```python
from build123d import *

# Parameters (mm, degrees)
EXTRUDE_1_DEPTH     = 10
EXTRUDE_2_DEPTH     = 120
CUT_EXTRUDE_1_DEPTH = 10
EXTRUDE_3_DEPTH     = 10
SKETCH_8_W          = 35
SKETCH_8_H          = 50
EXTRUDE_4_DEPTH     = 50


with BuildPart() as part:
    # 草图1 → 凸台-拉伸1 (new body)
    with BuildSketch(Plane.XY):
        with BuildLine():
            Line((30, 0), (120, 0))
            ThreePointArc((120, 0), (141.213203436, 8.786796564), (150, 30))
            Line((150, 30), (150, 120))
            ThreePointArc((150, 120), (141.213203436, 141.213203436), (120, 150))
            Line((120, 150), (30, 150))
            ThreePointArc((30, 150), (8.786796564, 141.213203436), (0, 120))
            Line((0, 120), (0, 30))
            ThreePointArc((0, 30), (8.786796564, 8.786796564), (30, 0))
        make_face()
    extrude(amount=EXTRUDE_1_DEPTH)

    # 草图2 → 凸台-拉伸2 (add)
    with BuildSketch(Plane.XY.offset(10)):
        with BuildLine():
            ThreePointArc((100, 75), (84.567085809, 98.096988313), (57.32233047, 92.67766953))
            Line((57.32233047, 92.67766953), (92.67766953, 57.32233047))
            ThreePointArc((92.67766953, 57.32233047), (98.096988313, 65.432914191), (100, 75))
        make_face()
        with BuildLine():
            Line((92.67766953, 57.32233047), (57.32233047, 92.67766953))
            ThreePointArc((57.32233047, 92.67766953), (57.32233047, 57.32233047), (92.67766953, 57.32233047))
        make_face()
    extrude(amount=EXTRUDE_2_DEPTH)

    # 草图5 → 切除-拉伸1 (cut)
    with BuildSketch(Plane.XY.offset(130)):
        with BuildLine():
            ThreePointArc((67.4, 86), (61.595836944, 88.404163056), (64, 82.6))
            Line((64, 82.6), (64, 86))
            Line((64, 86), (67.4, 86))
        make_face()
        with BuildLine():
            Line((64, 86), (64, 82.6))
            ThreePointArc((64, 82.6), (66.404163056, 83.595836944), (67.4, 86))
            Line((67.4, 86), (64, 86))
        make_face()
        with BuildLine():
            Line((64, 67.4), (64, 64))
            Line((64, 64), (67.4, 64))
            ThreePointArc((67.4, 64), (66.404163056, 66.404163056), (64, 67.4))
        make_face()
        with BuildLine():
            Line((67.4, 64), (64, 64))
            Line((64, 64), (64, 67.4))
            ThreePointArc((64, 67.4), (61.595836944, 61.595836944), (67.4, 64))
        make_face()
        with BuildLine():
            ThreePointArc((86, 67.4), (83.595836944, 66.404163056), (82.6, 64))
            Line((82.6, 64), (86, 64))
            Line((86, 64), (86, 67.4))
        make_face()
        with BuildLine():
            Line((86, 64), (82.6, 64))
            ThreePointArc((82.6, 64), (86, 60.6), (89.4, 64))
            ThreePointArc((89.4, 64), (88.404163056, 66.404163056), (86, 67.4))
            Line((86, 67.4), (86, 64))
        make_face()
        with BuildLine():
            ThreePointArc((82.6, 86), (83.595836944, 83.595836944), (86, 82.6))
            Line((86, 82.6), (86, 86))
            Line((86, 86), (82.6, 86))
        make_face()
        with BuildLine():
            Line((86, 86), (86, 82.6))
            ThreePointArc((86, 82.6), (88.404163056, 83.595836944), (89.4, 86))
            ThreePointArc((89.4, 86), (86, 89.4), (82.6, 86))
            Line((82.6, 86), (86, 86))
        make_face()
    extrude(amount=-CUT_EXTRUDE_1_DEPTH, mode=Mode.SUBTRACT)

    # 草图7 → 凸台-拉伸3 (add, through all)
    with BuildSketch(Plane.XY.offset(10)):
        Polygon((0, 102.5), (-35, 102.5), (-35, 47.5), (0, 47.5), (0, 75), align=None)
    extrude(amount=-EXTRUDE_3_DEPTH)

    # 草图8 → 凸台-拉伸4 (add)
    with BuildSketch(Plane.XY.offset(10)):
        Polygon((-35, 102.5), (0, 102.5), (5, 102.5), (5, 47.5), (0, 47.5), (-35, 47.5), align=None)
        with Locations((-15, 75)):
            Rectangle(SKETCH_8_W, SKETCH_8_H, mode=Mode.SUBTRACT)
    extrude(amount=EXTRUDE_4_DEPTH)


solid = part.part
```
Geometry: final body of the model. Coordinates: model frame, mm. A direction names the side the tool comes from. Round coordinates to 2 decimals unless told otherwise and drop trailing zeros. Loops run counter-clockwise (first coordinate to the right, second up) from the corner with the lowest first, then second, coordinate; pieces in that order, holes last.
Item 1: Section D-D, the plane z = 79.5. Output: boundary loops of the cut face in (x, y), plus the area to 3 significant figures.
Checked values:
outline: circle Ø50 at (75, 75)
area: 1,960 mm2
Item 2: Section B-B, the plane y = 95. Output: boundary loops of the cut face in (x, z).
Checked values:
outline: (-35, 0) - (150, 0) - (150, 10) - (90, 10) - (90, 130) - (60, 130) - (60, 10) - (5, 10) - (5, 60) - (2.5, 60) - (2.5, 10) - (-32.5, 10) - (-32.5, 60) - (-35, 60) - close
Item 3: Section A-A, the plane z = 57. Output: boundary loops of the cut face in (x, y), plus the area to 3 significant figures.
Checked values:
outline: (-35, 47.5) - (5, 47.5) - (5, 102.5) - (-35, 102.5) - close; circle Ø50 at (75, 75); hole (-32.5, 50) - (2.5, 50) - (2.5, 100) - (-32.5, 100) - close
area: 2,410 mm2
Item 4: Reachability of faces 1 (the flat face through (0, 111, 5)), 2 (the flat face through (76, 150, 5)), 3 (the flat face through (2.5, 75, 35)), 4 (the flat face through (0, 39, 5)) from +Z, -Z, +X, -X, +Y, -Y: full face, straight path, thin tool, end or side. Return the list, or none.
Checked values:
face 1: +Z, -Z, -X, +Y
face 2: +Z, -Z, +X, -X, +Y
face 3: +Z
face 4: +Z, -Z, -X, -Y
Item 5: Contact query for flat-ended pins moving along their axis: P1, Ø20, axis at x = -8, y = 67.5, coming from the +Z side; P2, Ø11, axis at y = 110, z = 3.5, coming from the -X side; P3, Ø2, axis at x = 64.5, y = 86.5, coming from the +Z side. Output: stop coordinate, or through.
Checked values:
P1: stops at z = 10
P2: stops at x = 0
P3: stops at z = 120
Item 6: Section C-C, the plane x = -19. Output: boundary loops of the cut face in (y, z).
Checked values:
outline: (47.5, 0) - (102.5, 0) - (102.5, 60) - (100, 60) - (100, 10) - (50, 10) - (50, 60) - (47.5, 60) - close
Item 7: Mould query, pull axis X, two halves, no side actions, for faces 5 (the flat face through (-15, 100, 35)), 6 (the cylindrical face through (9.021, 141.445, 4.93)), 7 (the flat face through (74, 0, 5)), 8 (the flat face through (150, 74, 5)). Classes: released by +X, released by -X, zero draft, split by the parting line, or undercut.
Checked values:
face 5: undercut
face 6: released by -X
face 7: zero draft
face 8: released by +X
Item 8: Line query: L1, parallel to Y at x = 64, z = 126.75; L2, parallel to X at y = 97.5, z = 34.5; L3, parallel to Z at x = 126.5, y = 132. Output: solid intervals per line, ascending.
Checked values:
L1: y = 52.55 to 60.6, 67.4 to 82.6, 89.4 to 97.45
L2: x = -35 to -32.5, 2.5 to 5, 64.1 to 85.9
L3: z = 0 to 10
